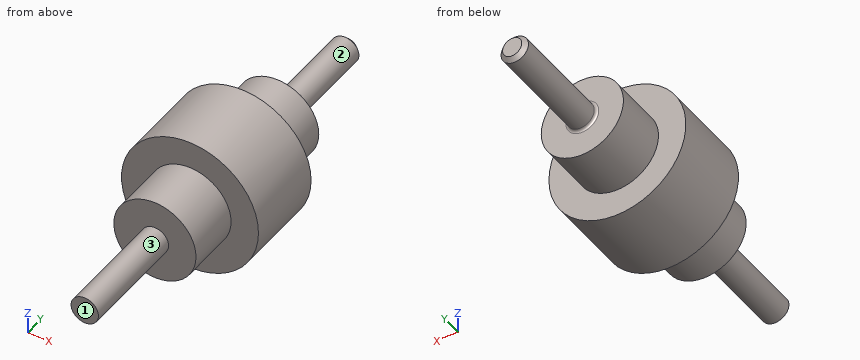
from build123d import *

# Parameters (mm, degrees)
F2_R    = 2
F3_SIZE = 3


with BuildPart() as f1:
    # F0 (on Top) → F1 (revolve)
    with BuildSketch(Plane.XY):
        Polygon((30, 55.720315), (10, 55.720315), (10, 135.720315), (0, 135.720315), (0, -164.279685), (10, -164.279685), (10, -84.279685), (30, -84.279685), (30, -44.279685), (50, -44.279685), (50, 15.720315), (30, 15.720315), align=None)
    revolve(axis=Axis((0, -14.279685, 0), (0, -1, 0)))

    # F2
    f2_edges = [f1.edges().sort_by_distance(p)[0] for p in [
        (-10, 55.720315, 0),
    ]]
    fillet(f2_edges, radius=F2_R)

    # F3
    f3_edges = [f1.edges().sort_by_distance(p)[0] for p in [
        (-10, 135.720315, 0),
    ]]
    chamfer(f3_edges, length=F3_SIZE)


solid = f1.part
Build history of the part. All positions in model axes, mm. Face numbers are marked on the shaded views. A direction names the side the tool comes from. Coordinates: 2 decimals unless noted, no trailing zeros. Write each loop counter-clockwise with the first axis right and the second up, starting at its lowest first coordinate (ties: lowest second). Pieces come first, ordered by that corner, then holes.
(1) Cut at B-B on x = 0. List the corners of the cut face in (y, z), and give its area (3 significant figures).
(2) 3-axis set-ups, long thin cutter, end or side, ignore diameter. For the marked faces 1, 2 and 3: which of +Z, -Z, +X, -X, +Y, -Y reach the whole face in a straight line?
(3) Drill centre lines: line 1 (Y direction, x = 4, z = 12); line 2 (Y direction, x = 42.5, z = 0); line 3 (Z direction, x = -1.5, y = 46.5). Where is each one in solid material? Low to high.
(4) Pin check, flat tips, straight feed: pin 1 Ø8 at (y, z) = (82.5, -7.5) entering from -X; pin 2 Ø10 at (x, z) = (-39.5, 32.5) entering from +Y; pin 3 Ø8 at (x, y) = (7, 56.5) entering from -Z. Stop position of each tip, or through.
(5) Cut at A-A on z = 0. List the corners of the cut face in (x, y), and give its area (3 significant figures).
(6) Cut at D-D on z = -16.5. List the corners of the cut face in (x, y), and give its area (3 significant figures).
(7) Cut at C-C on y = -70.5. List the corners of the cut face in (x, z).
Working result:
1. outline: (-164.28, -10) - (-84.28, -10) - (-84.28, -30) - (-44.28, -30) - (-44.28, -50) - (15.72, -50) - (15.72, -30) - (55.72, -30) - (55.72, -12) arc R2 cw to (57.72, -10) - (132.72, -10) - (135.72, -7) - (135.72, 7) - (132.72, 10) - (57.72, 10) arc R2 cw to (55.72, 12) - (55.72, 30) - (15.72, 30) - (15.72, 50) - (-44.28, 50) - (-44.28, 30) - (-84.28, 30) - (-84.28, 10) - (-164.28, 10) - close
1. area: 14,000 mm2
2. face 1: +Z, -Z, +X, -X, -Y
2. face 2: +Y
2. face 3: -Y
3. line 1: y = -84.28 to 55.72
3. line 2: y = -44.28 to 15.72
3. line 3: z = -29.96 to 29.96
4. pin 1: stops at x = -9.37
4. pin 2: stops at y = 15.72
4. pin 3: stops at z = -29.84
5. outline: (-50, -44.28) - (-30, -44.28) - (-30, -84.28) - (-10, -84.28) - (-10, -164.28) - (10, -164.28) - (10, -84.28) - (30, -84.28) - (30, -44.28) - (50, -44.28) - (50, 15.72) - (30, 15.72) - (30, 55.72) - (12, 55.72) arc R2 cw to (10, 57.72) - (10, 132.72) - (7, 135.72) - (-7, 135.72) - (-10, 132.72) - (-10, 57.72) arc R2 cw to (-12, 55.72) - (-30, 55.72) - (-30, 15.72) - (-50, 15.72) - close
5. area: 14,000 mm2
6. outline: (-47.2, -44.28) - (-25.05, -44.28) - (-25.05, -84.28) - (25.05, -84.28) - (25.05, -44.28) - (47.2, -44.28) - (47.2, 15.72) - (25.05, 15.72) - (25.05, 55.72) - (-25.05, 55.72) - (-25.05, 15.72) - (-47.2, 15.72) - close
6. area: 9,670 mm2
7. outline: circle Ø60 at (0, 0)
